Autodesk Inventor part; units mm, degrees
ref_plane "YZ Plane" through (0, 0, 0) normal (1, 0, 0) x (0, 1, 0)
ref_plane "XZ Plane" through (0, 0, 0) normal (0, 1, 0) x (-1, 0, 0)
ref_plane "XY Plane" through (0, 0, 0) normal (0, 0, 1) x (1, 0, 0)
ref_plane "Work Plane1" through (0, 0, 0) normal (0, 0, 1) x (1, 0, 0)
sketch "Sketch1" plane through (0, 0, 0) normal (0, 0, 1) x (1, 0, 0)
  circle A0 centre (-115, 0) radius 5
  circle A1 centre (-115, 0) radius 126
  point P0 (0, 0)
  dimension "d0" = 252
extrude "Extrusion1" add sketch "Sketch1" along normal blind 1.8 contours A0 | A1
sketch "Sketch2" plane through (-115, 0, 1.8) normal (0, 0, 1) x (1, 0, 0)
  circle A0 centre (-55, 95.2628) radius 1.6
  circle A1 centre (-55, -95.2628) radius 1.75
  circle A2 centre (110, 0) radius 1.6
  circle A3 centre (0, 0) radius 126
  line L0 (-55, 95.2628) -> (110, 0)
  line L1 (110, 0) -> (-55, -95.2628)
  line L2 (-55, -95.2628) -> (-55, 95.2628)
  point P0 (115, 0)
  dimension "d3" = 3.2
  dimension "d4" = 3.5
  dimension "d5" = 3.2
  dimension "d11" = 110
extrude "Extrusion2" cut sketch "Sketch2" against normal blind 10 contours A0 L0 L2 | L2 L0 A0 | L2 L1 A1 | A1 L1 L2 | L0 L1 A2 | A2 L1 L0
chamfer "Chamfer1" distance 1.7 angle 45 3 edges at (-6.6, 0, 1.8) (-171.6, 95.2628, 1.8) (-171.75, -95.2628, 1.8)
sketch "Sketch3" plane through (-115, 0, 1.8) normal (0, 0, 1) x (1, 0, 0)
  circle A0 centre (0, 0) radius 126
  line L0 (-1, -129) -> (-5.9628, -131.8653)
  line L1 (1, -129) -> (5.9628, -131.8653)
  arc A1 (6.0472, -127.8571) -> (5.9528, -125.8593) centre (6, -126.8582) ccw
  arc A2 (-5.9528, -125.8593) -> (-6.0472, -127.8571) centre (-6, -126.8582) ccw
  line L2 (13.7031, -128.2781) -> (16.5283, -124.9112)
  line L3 (-13.7031, -128.2781) -> (-16.5283, -124.9112)
  arc A3 (-6.538, -131.838) -> (-5.9628, -131.8653) centre (0, 0) ccw
  arc A4 (5.9628, -131.8653) -> (6.538, -131.838) centre (0, 0) ccw
  line L4 (1, -127.9961) -> (1, -129)
  line L5 (-1, -127.9961) -> (-1, -129)
  arc A5 (-6.0472, -127.8571) -> (-1, -127.9961) centre (0, 0) ccw
  arc A6 (1, -127.9961) -> (6.0472, -127.8571) centre (0, 0) ccw
  arc A7 (-13.7031, -128.2781) -> (-6.538, -131.838) centre (-6.0427, -121.8503) ccw
  arc A8 (6.538, -131.838) -> (13.7031, -128.2781) centre (6.0427, -121.8503) ccw
  point P0 (115, 0)
  point P1 (10.9628, -131.544)
  point P2 (-10.9628, -131.544)
  dimension "d17" = 129
  dimension "d18" = 129
  dimension "d23" = 5
  dimension "d25" = 5
  dimension "d28" = 10
extrude "Extrusion3" add sketch "Sketch3" against normal up to surface (1.8 mm away) contours A0 A2 A5 L5 L0 A3 A7 L3 | L2 A8 A4 L1 L4 A6 A1 A0
fillet "Fillet1" radius 5 4 edges at (-109.0372, -131.8653, 0.9) (-120.9628, -131.8653, 0.9) (-131.5283, -124.9112, 0.9) (-98.4717, -124.9112, 0.9)
sketch "Sketch4" plane through (0, 0, 0) normal (0, 0, -1) x (-1, 0, 0)
  arc A0 (133.3939, -124.6502) -> (96.6061, -124.6502) centre (115, 0) ccw
  arc A1 (116, -127.9961) -> (121.0472, -127.8571) centre (115, 0) ccw
  line L0 (115, 0) -> (252.9222, 0) construction
  line L1 (209.3241, 52.4043) -> (223.0286, 58.5024)
  line L2 (229.1267, 44.7979) -> (215.4222, 38.6998)
  line L3 (209.3241, 52.4043) -> (229.1267, 44.7979) construction
  line L4 (223.0286, 58.5024) -> (215.4222, 38.6998) construction
  line L5 (211.6138, 47.2585) -> (225.2106, 53.5988)
  line L6 (223.0286, 58.5024) -> (225.2106, 53.5988)
  line L7 (226.0238, 51.7712) -> (229.1267, 44.7979)
  line L8 (215.4222, 38.6998) -> (212.427, 45.431)
  line L9 (211.6138, 47.2585) -> (209.3241, 52.4043)
  line L10 (115, 0) -> (226.0238, 51.7712)
  point P0 (0, 0)
  point P1 (219.2254, 48.6011)
  dimension "d34" = 15
  dimension "d36" = 115
extrude "Extrusion4" add sketch "Sketch4" along normal blind 1
properties material "Aluminum 6061"
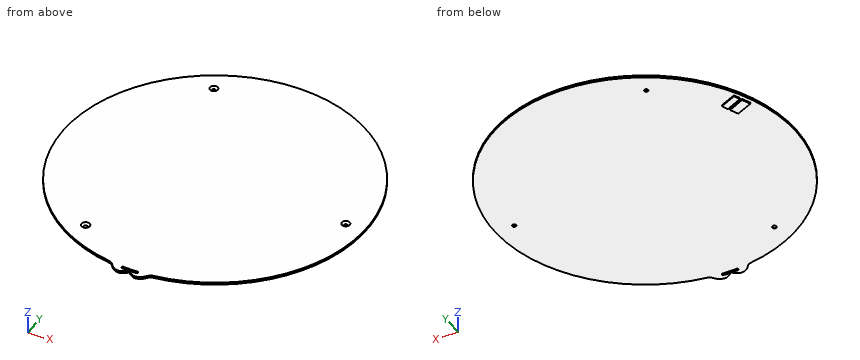
The model under review builds one solid part; all positions refer to its coordinate system, in mm. Round coordinates to 2 decimals unless told otherwise and drop trailing zeros. Loops run counter-clockwise (first coordinate to the right, second up) from the corner with the lowest first, then second, coordinate; pieces in that order, holes last. Notation, with made-up numbers: (-20, 25.5) -> (11, 25.5) arc R12 cw to (11, 37.5) -> close; hole circle Ø1 at (64, 55). An arc over 180 degrees is marked (long way). Answer as CSV lines item,"result".
1) For P1, Ø1, axis at y = -2, z = 1.5, coming from the -X side; P2, Ø1.5, axis at x = -171, y = 48, coming from the -Z side; P3, Ø0.5, axis at y = -128.5, z = 1, coming from the +X side; P4, Ø3, axis at x = -170, y = 95.26, coming from the +Z side, all flat-tipped, find the tip position at first contact; note any pin that passes through.
Geometry results:
P1,"stops at x = -240.99"
P2,"stops at z = 0"
P3,"stops at x = -101.27"
P4,"passes through"
2) Add section A-A on z = -0.5. Write out the cut boundary in (x, y), plus the area to 3 significant figures.
Geometry results:
outline,"(-229.13, 44.8) -> (-215.42, 38.7) -> (-212.43, 45.43) -> (-226.02, 51.77) -> close; (-225.21, 53.6) -> (-211.61, 47.26) -> (-209.32, 52.4) -> (-223.03, 58.5) -> close"
area,"195 mm²"
3) Add section B-B on x = -86.5. Write out the cut boundary in (y, z).
Geometry results:
outline,"(-122.73, 0) -> (122.73, 0) -> (122.73, 1.8) -> (-122.73, 1.8) -> close"
4) Add section C-C on y = 69. Write out the cut boundary in (x, z).
Geometry results:
outline,"(-220.43, 0) -> (-9.57, 0) -> (-9.57, 1.8) -> (-220.43, 1.8) -> close"
5) To check wall thickness, follow line 1 along Y through (x, z) = (-170, 0.1); line 2 along Z through (x, y) = (-119.5, -5.5); line 3 along X through (y, z) = (-2, 0.45). State the ranges of each line that lie inside material, in increasing order. Write a range as from..to.
Geometry results:
line 1,"y = -113.36..-97.01, -93.51..93.66, 96.86..113.36"
line 2,"z = 0..1.8"
line 3,"x = -240.98..10.98"
